Work out the finished part from the listing and answer in its coordinate system (mm). Give positions to 0.01 mm unless a question says otherwise; leave off trailing zeros. Loops run counter-clockwise (first coordinate to the right, second up) from the corner with the lowest first, then second, coordinate; pieces in that order, holes last. Notation, with made-up numbers: M 4.25,0 L 29.25,0 A32 ccw 29.25,31 Z; hole C 10,-17 d11. An arc over 180 degrees is marked long. Write item = value, one per line. Start each with the question number.
1. Flat-ended cylindrical pins translate along their axes: pin 1 Ø1 at (y, z) = (-53, -3) entering from -X; pin 2 Ø1 at (x, z) = (-42, -1.5) entering from -Y. Find the tip coordinate at first contact, or state that the pin passes through.
2. Section D-D on y = -23 is taken. Determine the outline of the cut face in (x, z), plus the area to 3 significant figures.
3. Section B-B on x = -8.5 is taken. Determine the outline of the cut face in (y, z), plus the area to 3 significant figures.
4. Section A-A on y = -51.5 is taken. Determine the outline of the cut face in (x, z).
5. Consider L1, parallel to Y at x = -8, z = -1.6; L2, parallel to X at y = -60.5, z = -0.4; L3, parallel to Y at x = -40, z = -2.8. Determine where each line is inside the solid, lowest interval first. Write a range as [from, to].
6. Section C-C on z = -0.95 is taken. Determine the outline of the cut face in (x, y).
7. The mould has two halves that part along X. Classify faces 1 (the face through (-57, -55, -3.404)), 2 (the face through (6.8, -18.47, -1.68)), 3 (the face through (0.034, -69.615, -1.678)): released by +X, released by -X, zero draft, split by the parting line, or undercut.
```python
from build123d import *

# Parameters (mm, degrees)
BOSS_EXTRUDE1_DEPTH             = 3.4036
F_1_4_CLEARANCE_HOLE1_D         = 6.7564
M4_CLEARANCE_HOLE1_D            = 4.5
HOLE_FOR_1_4_300_SC_NUTS_SP_1_D = 8.7376


with BuildPart() as part:
    # Sketch1 → Boss-Extrude1 (new body)
    with BuildSketch(Plane.XY):
        with BuildLine():
            Line((7.348321245, -20.048772414), (7.348321245, -67.889857088))
            ThreePointArc((7.348321245, -67.889857088), (6.372101393, -69.891404403), (4.193839631, -70.354408233))
            Line((4.193839631, -70.354408233), (2.419218956, -69.911945605))
            ThreePointArc((2.419218956, -69.911945605), (0, -69.614902867), (-2.419218956, -69.911945605))
            Line((-2.419218956, -69.911945605), (-103.101990119, -95.014979859))
            ThreePointArc((-103.101990119, -95.014979859), (-110.671589825, -93.883695604), (-115.224166338, -87.731241553))
            Line((-115.224166338, -87.731241553), (-122.84470605, -57.166926175))
            ThreePointArc((-122.84470605, -57.166926175), (-121.713421794, -49.59732647), (-115.560967743, -45.044749956))
            Line((-115.560967743, -45.044749956), (-2.419218956, -16.835343693))
            ThreePointArc((-2.419218956, -16.835343693), (0, -16.538300956), (2.419218956, -16.835343693))
            Line((2.419218956, -16.835343693), (5.42280286, -17.584221269))
            ThreePointArc((5.42280286, -17.584221269), (6.80986856, -18.484992267), (7.348321245, -20.048772414))
        make_face()
    extrude(amount=-BOSS_EXTRUDE1_DEPTH)

    # 1/4 Clearance Hole1 (through all)
    with Locations(Plane.XY):
        with Locations((-74.335136024, -53.317040996)):
            Hole(F_1_4_CLEARANCE_HOLE1_D / 2)

    # M4 Clearance Hole1 (through all)
    with Locations(Plane.XY):
        with Locations((-110.721225759, -62.389112081), (-37.949046288, -44.244969911)):
            Hole(M4_CLEARANCE_HOLE1_D / 2)

    # Hole for 1/4 300® SC Nuts (SP)1 (through all)
    with Locations(Plane.XY):
        with Locations((-7.366, -61.569560235), (-7.366, -29.819560235)):
            Hole(HOLE_FOR_1_4_300_SC_NUTS_SP_1_D / 2)


solid = part.part
```
Verdict:
q1.pin_1 = -123.06
q1.pin_2 = -79.91
q2.outline = M -27.14,-3.4 L 7.35,-3.4 L 7.35,0 L -27.14,0 Z
q2.area = 117 mm2
q3.outline = M -71.43,-3.4 L -65.79,-3.4 L -65.79,0 L -71.43,0 Z; M -57.35,-3.4 L -34.04,-3.4 L -34.04,0 L -57.35,0 Z; M -25.6,-3.4 L -18.35,-3.4 L -18.35,0 L -25.6,0 Z
q3.area = 123 mm2
q4.outline = M -122.6,-3.4 L -77.18,-3.4 L -77.18,0 L -122.6,0 Z; M -71.49,-3.4 L 7.35,-3.4 L 7.35,0 L -71.49,0 Z
q5.L1 = [-71.3, -65.89], [-57.25, -34.14], [-25.5, -18.23]
q5.L2 = [-122.01, -111.94], [-109.5, -11.6], [-3.13, 7.35]
q5.L3 = [-79.28, -45.17], [-43.32, -26.21]
q6.outline = M -122.84,-57.17 L -115.22,-87.73 A10 ccw -103.1,-95.01 L -2.42,-69.91 A10 cw 2.42,-69.91 L 4.19,-70.35 A2.54 ccw 7.35,-67.89 L 7.35,-20.05 A2.54 ccw 5.42,-17.58 L 2.42,-16.84 A10 ccw -2.42,-16.84 L -115.56,-45.04 A10 ccw Z; hole C -110.72,-62.39 d4.5; hole C -74.34,-53.32 d6.76; hole C -37.95,-44.24 d4.5; hole C -7.37,-61.57 d8.74; hole C -7.37,-29.82 d8.74
q7.face_1 = zero draft
q7.face_2 = released by +X
q7.face_3 = undercut
